Autodesk Inventor part; units mm, degrees
ref_plane "YZ Plane" through (0, 0, 0) normal (1, 0, 0) x (0, 1, 0)
ref_plane "XZ Plane" through (0, 0, 0) normal (0, 1, 0) x (-1, 0, 0)
ref_plane "XY Plane" through (0, 0, 0) normal (0, 0, 1) x (1, 0, 0)
sketch "スケッチ1" plane through (0, 0, 0) normal (0, 0, 1) x (1, 0, 0)
  line L0 (0, 0) -> (8.2, 0)
  line L1 (8.2, 0) -> (4.1, 0)
  line L2 (0, 0) -> (0, 12)
  line L3 (8.2, 0) -> (8.2, 12)
  line L4 (4.1, 0) -> (4.1, 9.65)
  line L5 (0, 12) -> (1.1, 12)
  line L6 (8.2, 12) -> (7.1, 12)
  arc A0 (1.1, 12) -> (7.1, 12) centre (4.1, 12.7399) ccw
  dimension "d0" = 8.2
  dimension "d1" = 12
  dimension "d2" = 12
  dimension "d3" = 9.65
  dimension "d4" = 1.1
  dimension "d5" = 1.1
revolve "回転1" add sketch "スケッチ1" angle 360 about axis through (0, 0, 0) along (1, 0, 0)
sketch "スケッチ2" plane through (8.2, 0, 0) normal (1, 0, 0) x (0, 0, -1)
  circle A0 centre (0, 0) radius 12
  line L0 (0, 0) -> (22.8, 0)
  line L1 (0, 0) -> (0, -7.2)
  line L2 (0, 0) -> (22.8, 0)
  line L3 (22.8, 0) -> (22.8, -7.2)
  line L4 (22.8, -7.2) -> (0, -7.2)
  line L5 (0, -7.2) -> (0, 0)
  line L6 (0, 0) -> (-22.8, 0)
  line L7 (-22.8, 0) -> (-22.8, -7.2)
  line L8 (-22.8, -7.2) -> (0, -7.2)
  dimension "d7" = 22.8
  dimension "d8" = 7.2
  dimension "d17" = 0
extrude "押し出し1" add sketch "スケッチ2" along normal blind 1.2 contours L0 L3 L4 A0 | A0 L4 L1 L0 | L6 L1 L8 A0 | A0 L8 L7 L6
sketch "スケッチ3" plane through (0, 0, 0) normal (-1, 0, 0) x (0, 0, 1)
  circle A0 centre (0, 0) radius 12
  line L0 (0, 0) -> (0, -7.2)
  line L1 (0, -7.2) -> (22.8, -7.2)
  line L2 (0, 0) -> (22.8, 0)
  line L3 (22.8, 0) -> (22.8, -7.2)
  line L4 (22.8, -7.2) -> (0, -7.2)
  line L5 (0, -7.2) -> (0, 0)
  line L6 (0, 0) -> (-22.8, 0)
  line L7 (-22.8, 0) -> (-22.8, -7.2)
  line L8 (-22.8, -7.2) -> (0, -7.2)
  dimension "d11" = 7.2
  dimension "d12" = 22.8
extrude "押し出し2" add sketch "スケッチ3" along normal blind 2 contours L2 L3 L1 A0 | A0 L1 L0 L2 | L6 L0 L8 A0 | A0 L8 L7 L6
sketch "スケッチ4" plane through (-2, 0, 0) normal (-1, 0, 0) x (0, 0, 1)
  line L0 (-22.8, -7.2) -> (22.8, -7.2)
  line L1 (0, -7.2) -> (12.1, -7.2)
  line L2 (12.1, -7.2) -> (30.2, -7.2)
  line L3 (12.1, -7.2) -> (30.2, -7.2)
  line L4 (30.2, -7.2) -> (30.2, -8.4)
  line L5 (30.2, -8.4) -> (12.1, -8.4)
  line L6 (12.1, -8.4) -> (12.1, -7.2)
  line L7 (0, 0) -> (0, -1.8874)
  line L8 (-12.1, -7.2) -> (-30.2, -7.2)
  line L9 (-30.2, -7.2) -> (-30.2, -8.4)
  line L10 (-30.2, -8.4) -> (-12.1, -8.4)
  line L11 (-12.1, -8.4) -> (-12.1, -7.2)
  dimension "d15" = 12.1
  dimension "d16" = 18.1
  dimension "d18" = 1.2
extrude "押し出し3" add sketch "スケッチ4" against normal blind 12
sketch "スケッチ5" plane through (-2, -8.4, 12.1) normal (0, -1, 0) x (1, 0, 0)
  line L0 (0, 18.1) -> (12, 18.1)
  line L1 (6, 18.1) -> (6, 13.4)
  line L2 (6, 13.4) -> (6, -37.2)
  circle A0 centre (6, -37.2) radius 1.6
  circle A1 centre (6, 13.4) radius 1.6
  point P0 (2, -12.1)
  dimension "d21" = 4.7
  dimension "d22" = 50.6
  dimension "d23" = 3.2
  dimension "d24" = 3.2
hole "穴1" at (4, -8.4, 25.5) at (4, -8.4, -25.1) direction (0, 1, 0) diameter 3.2 depth 8 tip angle 118
properties part number "知能ロボコンショウレックス戸草"
Check sheet for the modelled part. Datum: model origin and axes. Units: mm. A direction names the side the tool comes from. Coordinates: 2 decimals unless noted, no trailing zeros. Write each loop counter-clockwise with the first axis right and the second up, starting at its lowest first coordinate (ties: lowest second). Pieces come first, ordered by that corner, then holes. Notation, with made-up numbers: (43.25, -36) -> (72.25, -36) arc R11 ccw to (72.25, -18) -> close; hole circle Ø2 at (52.5, -9.5). An arc over 180 degrees is marked (long way). Use a Markdown table: item, result.
1. Tool access check on faces 1 (the flat face through (-1, 0, 0)), 2 (the flat face through (9, -7.2, 0)), 3 (the cylindrical face through (0.56, -11.99, 0.53)), 4 (the flat face through (-1, -4, -22.8)), 5 (the flat face through (0, -4, -16)). Record the directions out of +Z, -Z, +X, -X, +Y, -Y that give a thin tool (end or side, any length) a straight path to the whole face; none if there is none.
Reported:
| item | result |
|---|---|
| face 1 | +Z, -Z, -X, +Y |
| face 2 | +X, -Y |
| face 3 | none |
| face 4 | -Z, +X, -X, +Y |
| face 5 | -Z |
2. Sectioned sample at B-B (z = -25.1). Enter the section's corners in (x, y).
Reported:
| item | result |
|---|---|
| outline | (-2, -8.4) -> (2.4, -8.4) -> (2.4, -7.2) -> (-2, -7.2) -> close; (5.6, -8.4) -> (10, -8.4) -> (10, -7.2) -> (5.6, -7.2) -> close |
3. Go/stop test with flat-tipped pins: pin 1 Ø13 at (y, z) = (7.5, 6) entering from +X; pin 2 Ø3.5 at (x, z) = (2.5, 24.5) entering from +Y; pin 3 Ø6 at (x, z) = (4, 22.5) entering from -Y; pin 4 Ø1.9 at (x, z) = (4, 25.5) entering from -Y. Record where each tip stops, or that it passes through.
Reported:
| item | result |
|---|---|
| pin 1 | stops at x = 8.2 |
| pin 2 | stops at y = -7.2 |
| pin 3 | stops at y = -8.4 |
| pin 4 | passes through |
4. Sectioned sample at C-C (z = 0). Enter the section's corners in (x, y).
Reported:
| item | result |
|---|---|
| outline | (-2, -7.2) -> (0, -7.2) -> (0, -12) -> (1.1, -12) arc R3.09 cw to (7.1, -12) -> (8.2, -12) -> (8.2, -7.2) -> (9.4, -7.2) -> (9.4, 0) -> (8.2, 0) -> (8.2, 12) -> (7.1, 12) arc R3.09 cw to (1.1, 12) -> (0, 12) -> (0, 0) -> (-2, 0) -> close |
5. Sectioned sample at A-A (x = 3). Enter the section's corners in (y, z), plus the area to 3 significant figures.
Reported:
| item | result |
|---|---|
| outline | circle Ø19.7 at (0, 0); (-8.4, -30.2) -> (-7.2, -30.2) -> (-7.2, -26.35) -> (-8.4, -26.35) -> close; (-8.4, -23.85) -> (-7.2, -23.85) -> (-7.2, -12.1) -> (-8.4, -12.1) -> close; (-8.4, 12.1) -> (-7.2, 12.1) -> (-7.2, 24.25) -> (-8.4, 24.25) -> close; (-8.4, 26.75) -> (-7.2, 26.75) -> (-7.2, 30.2) -> (-8.4, 30.2) -> close |
| area | 342 mm2 |
6. Release check for a two-part mould opening along Z. For faces 6 (the flat face through (4, -8, -12.1)), 7 (the flat face through (-1, -4, 22.8)), 8 (the flat face through (4, -8, -30.2)) record: pulls with the +Z half, pulls with the -Z half, needs draft (parallel to the pull), parting line crosses it, or undercut.
Reported:
| item | result |
|---|---|
| face 6 | undercut |
| face 7 | pulls with the +Z half |
| face 8 | pulls with the -Z half |
7. Scan lines: line 1 along X through (y, z) = (-4, -12.5); line 2 along Z through (x, y) = (4, -7.95); line 3 along Z through (x, y) = (4, -7.5). Record each from-to range of solid material in increasing order.
Reported:
| item | result |
|---|---|
| line 1 | x = -2 to 0, 8.2 to 9.4 |
| line 2 | z = -30.2 to -26.7, -23.5 to -12.1, -5.47 to 5.47, 12.1 to 23.9, 27.1 to 30.2 |
| line 3 | z = -30.2 to -26.7, -23.5 to -12.1, -6.07 to 6.07, 12.1 to 23.9, 27.1 to 30.2 |
